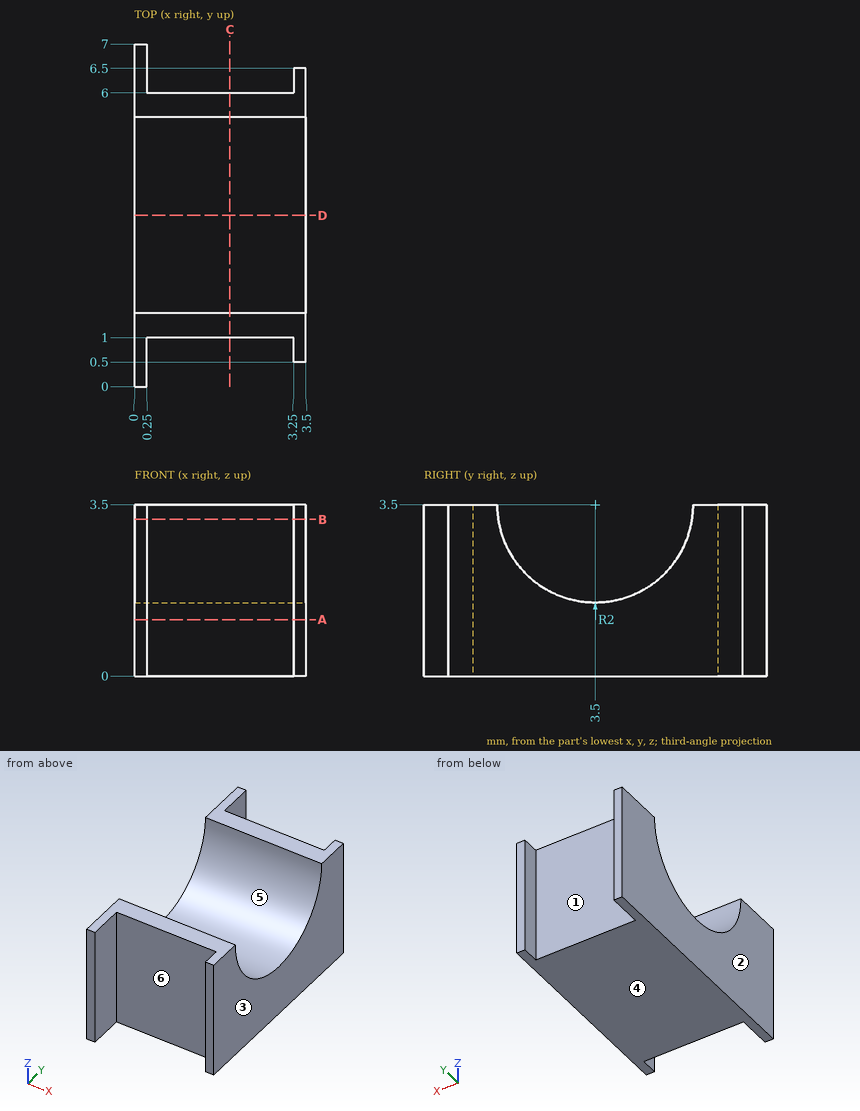
Verification items for this drawing (mm, ordinates from the low corner). A direction names the side the tool comes from. Give positions to 0.01 mm unless a question says otherwise; leave off trailing zeros. Write each loop counter-clockwise with the first axis right and the second up, starting at its lowest first coordinate (ties: lowest second). Pieces come first, ordered by that corner, then holes. Notation, with made-up numbers: (60.25, 47.25) -> (94.25, 47.25) arc R22 ccw to (94.25, 82.25) -> close; hole circle Ø11 at (12, -16.75). An arc over 180 degrees is marked (long way). Use CSV: the item, a comma, the result in double quotes. Start each with the question number.
Q1. Depth check by flat-ended pin: P1, Ø1, axis at x = 3, z = 1, coming from the +Y side; P2, Ø1.5, axis at x = 2, z = 1, coming from the +Y side; P3, Ø0.9, axis at x = 1.5, z = 2.5, coming from the -Y side; P4, Ø1, axis at x = 0.5, y = 2, coming from the -Z side. Enter the tip coordinate at first touch or a pass-through.
Q2. Scan lines: line 1 along Y through (x, z) = (2.7, 2.55); line 2 along Y through (x, z) = (1.5, 0.55); line 3 along Y through (x, z) = (0.55, 1.95). Record each from-to range of solid material in increasing order.
Q3. Release check for a two-part mould opening along X. For the marked faces 1, 2, 3 and 4 record: +X half, -X half, draft (parallel to the pull), parting line (faces both ways), or undercut.
Q4. Cross-section at C-C on x = 1.95. Enter the section's corners in (y, z).
Q5. Cross-section at D-D on y = 3.5. Enter the section's corners in (x, z).
Q6. Cross-section at B-B on z = 3.2. Enter the section's corners in (x, y).
Q7. Cross-section at A-A on z = 1.15. Enter the section's corners in (x, y), and give its area (4 significant figures).
Q8. Tool access check on the marked faces 5 and 6. Record the directions out of +Z, -Z, +X, -X, +Y, -Y that give a thin tool (end or side, any length) a straight path to the whole face; none if there is none.
Working result:
1,P1,"stops at y = 6.5"
1,P2,"stops at y = 6"
1,P3,"stops at y = 1"
1,P4,"stops at z = 0"
2,line 1,"y = 1 to 1.74, 5.26 to 6"
2,line 2,"y = 1 to 6"
2,line 3,"y = 1 to 2.24, 4.76 to 6"
3,face 1,"undercut"
3,face 2,"-X half"
3,face 3,"+X half"
3,face 4,"draft"
4,outline,"(1, 0) -> (6, 0) -> (6, 3.5) -> (5.5, 3.5) arc R2 cw to (1.5, 3.5) -> (1, 3.5) -> close"
5,outline,"(0, 0) -> (3.5, 0) -> (3.5, 1.5) -> (0, 1.5) -> close"
6,outline,"(0, 0) -> (0.25, 0) -> (0.25, 1) -> (3.25, 1) -> (3.25, 0.5) -> (3.5, 0.5) -> (3.5, 1.52) -> (0, 1.52) -> close; (0, 5.48) -> (3.5, 5.48) -> (3.5, 6.5) -> (3.25, 6.5) -> (3.25, 6) -> (0.25, 6) -> (0.25, 7) -> (0, 7) -> close"
7,outline,"(0, 0) -> (0.25, 0) -> (0.25, 1) -> (3.25, 1) -> (3.25, 0.5) -> (3.5, 0.5) -> (3.5, 6.5) -> (3.25, 6.5) -> (3.25, 6) -> (0.25, 6) -> (0.25, 7) -> (0, 7) -> close"
7,area,"18.25 mm^2"
8,face 5,"+Z, +X, -X"
8,face 6,"+Z, -Z, -Y"
